```python
from build123d import *

# Parameters (mm, degrees)
BOSS_EXTRUDE1_DEPTH = 10
SKETCH3_W           = 65
SKETCH3_H           = 37
BOSS_EXTRUDE2_DEPTH = 2
SKETCH4_R           = 1.5
CUT_EXTRUDE1_DEPTH  = 5


with BuildPart() as part:
    # Sketch2 → Boss-Extrude1 (new body)
    with BuildSketch(Plane.XY):
        Polygon((-17.5, 0), (-17.5, -1), (-14.5, -1), (-14.5, -5), (-22.5, -5), (-22.5, 0), (-22.5, 4), (22.5, 4), (22.5, -5), (14.5, -5), (14.5, -1), (17.5, -1), (17.5, 0), align=None)
    extrude(amount=BOSS_EXTRUDE1_DEPTH)

    # Sketch3 → Boss-Extrude2 (add)
    with BuildSketch(Plane(origin=(0, 4, 0), x_dir=(1, 0, 0), z_dir=(0, 1, 0))):
        with Locations((0, -5)):
            Rectangle(SKETCH3_W, SKETCH3_H)
    extrude(amount=BOSS_EXTRUDE2_DEPTH)

    # Sketch4 → Cut-Extrude1 (cut)
    with BuildSketch(Plane(origin=(0, 6, 0), x_dir=(1, 0, 0), z_dir=(0, 1, 0))):
        with Locations((-29.25, 8)):
            Circle(SKETCH4_R)
        with Locations((-29.25, -18)):
            Circle(SKETCH4_R)
        with Locations((29.25, -18)):
            Circle(SKETCH4_R)
        with Locations((29.25, 8)):
            Circle(SKETCH4_R)
    extrude(amount=-CUT_EXTRUDE1_DEPTH, mode=Mode.SUBTRACT)


solid = part.part
```
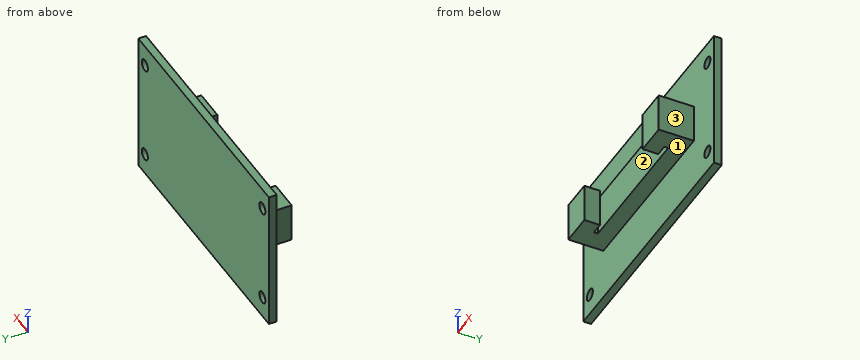
The model under review builds one solid part; all positions refer to its coordinate system, in mm. Face numbers are marked on the shaded views. Coordinates: 2 decimals unless noted, no trailing zeros. Loops run counter-clockwise (first coordinate to the right, second up) from the corner with the lowest first, then second, coordinate; pieces in that order, holes last. Notation, with made-up numbers: (21.5, 83.5) -> (66.5, 83.5) arc R16 cw to (66.5, 99.5) -> close; hole circle Ø5 at (29.25, 60.25). An arc over 180 degrees is marked (long way). Answer as CSV lines item,"result".
Item 1: Take a section at A-A, the plane z = 18. State the section outline as (x, y) points, and give its area (3 significant figures).
Results below:
outline,"(-32.5, 4) -> (-30.75, 4) -> (-30.75, 6) -> (-32.5, 6) -> close; (-27.75, 4) -> (27.75, 4) -> (27.75, 6) -> (-27.75, 6) -> close; (30.75, 4) -> (32.5, 4) -> (32.5, 6) -> (30.75, 6) -> close"
area,"118 mm2"
Item 2: Draft analysis for pull direction X (two halves, no side actions). For the marked faces 1, 2 and 3, state which applies: +X half, -X half, draft (parallel to the pull), parting line (faces both ways), or undercut.
Results below:
face 1,"draft"
face 2,"undercut"
face 3,"+X half"
Item 3: Insertion check: pin 1 (1.1 mm diameter, centred on y = -0.5, z = 6, fed in from -X); pin 2 (4.5 mm diameter, centred on y = -1, z = 6, fed in from +X); pin 3 (2.5 mm diameter, centred on x = 6.5, y = 0.5, fed in from +Z). Each pin has a flat end and moves straight along its axis. Give the tip position at first contact, or say it passes through.
Results below:
pin 1,"stops at x = -22.5"
pin 2,"stops at x = 22.5"
pin 3,"stops at z = 10"
Item 4: For L1, parallel to Z at x = -29.25, y = 5.2; L2, parallel to X at y = 5.4, z = 18; L3, parallel to X at y = -2.5, z = 1.5, list the stretches that pass through material, from the lowest coordinate up.
Results below:
L1,"z = -13.5 to -9.5, -6.5 to 16.5, 19.5 to 23.5"
L2,"x = -32.5 to -30.75, -27.75 to 27.75, 30.75 to 32.5"
L3,"x = -22.5 to -14.5, 14.5 to 22.5"
Item 5: Take a section at D-D, the plane x = -5. State the section outline as (y, z) points.
Results below:
outline,"(0, 0) -> (4, 0) -> (4, -13.5) -> (6, -13.5) -> (6, 23.5) -> (4, 23.5) -> (4, 10) -> (0, 10) -> close"
Item 6: Take a section at B-B, the plane x = 29.25. State the section outline as (y, z) points, and give its area (3 significant figures).
Results below:
outline,"(4, -13.5) -> (6, -13.5) -> (6, -9.5) -> (4, -9.5) -> close; (4, -6.5) -> (6, -6.5) -> (6, 16.5) -> (4, 16.5) -> close; (4, 19.5) -> (6, 19.5) -> (6, 23.5) -> (4, 23.5) -> close"
area,"62.0 mm2"
Item 7: Take a section at C-C, the plane z = 4. State the section outline as (x, y) points.
Results below:
outline,"(-32.5, 4) -> (-22.5, 4) -> (-22.5, -5) -> (-14.5, -5) -> (-14.5, -1) -> (-17.5, -1) -> (-17.5, 0) -> (17.5, 0) -> (17.5, -1) -> (14.5, -1) -> (14.5, -5) -> (22.5, -5) -> (22.5, 4) -> (32.5, 4) -> (32.5, 6) -> (-32.5, 6) -> close"
